```python
from build123d import *

# Parameters (mm, degrees)
SKETCH1_R           = 3
BOSS_EXTRUDE1_DEPTH = 54
SKETCH2_R           = 3
BOSS_EXTRUDE2_DEPTH = 35.293714059
SKETCH3_R           = 3
BOSS_EXTRUDE3_DEPTH = 6
BOSS_EXTRUDE4_START = 6
SKETCH4_R           = 3
BOSS_EXTRUDE4_DEPTH = 6


with BuildPart() as part:
    # Sketch1 → Boss-Extrude1 (new body)
    with BuildSketch(Plane(origin=(0, 0, 0), x_dir=(1, 0, 0), z_dir=(0, 1, 0))):
        with Locations(Location((0, 0, 0), (0, 0, 270))):
            Circle(SKETCH1_R)
    extrude(amount=BOSS_EXTRUDE1_DEPTH)

    # Sketch2 → Boss-Extrude2 (add)
    with BuildSketch(Plane(origin=(0, 54, 0), x_dir=(1, 0, 0), z_dir=(0, 1, 0))):
        with Locations(Location((0, 0, 0), (0, 0, 270))):
            Circle(SKETCH2_R)
    extrude(amount=BOSS_EXTRUDE2_DEPTH)

    # Sketch3 → Boss-Extrude3 (add)
    with BuildSketch(Plane(origin=(0, 89.293714059, 0), x_dir=(1, 0, 0), z_dir=(0, 1, 0))):
        with Locations(Location((0, 0, 0), (0, 0, 270))):
            Circle(SKETCH3_R)
    extrude(amount=BOSS_EXTRUDE3_DEPTH)

    # Sketch4 → Boss-Extrude4 (add)
    with BuildSketch(Plane.XZ.offset(BOSS_EXTRUDE4_START)):
        with Locations(Location((0, 0, 0), (0, 0, 270))):
            Circle(SKETCH4_R)
    extrude(amount=-BOSS_EXTRUDE4_DEPTH)


solid = part.part
```
Check sheet for the modelled part. Datum: model origin and axes. Units: mm. Give positions to 0.01 mm unless a question says otherwise; leave off trailing zeros. Loops run counter-clockwise (first coordinate to the right, second up) from the corner with the lowest first, then second, coordinate; pieces in that order, holes last. Notation, with made-up numbers: M 75,48 L 124,48 A23 cw 124,86 Z; hole C 27,-26.5 d7. An arc over 180 degrees is marked long. Answer as CSV lines item,"result".
Item 1: Scan lines: L1, parallel to Z at x = 0.1, y = 38; L2, parallel to Z at x = 1.15, y = 64.5; L3, parallel to X at y = 48, z = 0.55. Record each from-to range of solid material in increasing order.
Reply:
L1,"-3 to 3"
L2,"-2.77 to 2.77"
L3,"-2.95 to 2.95"
Item 2: Sectioned sample at A-A, the plane y = 65. Enter the section's corners in (x, z).
Reply:
outline,"C 0,0 d6"
Item 3: Depth check by flat-ended pin: pin 1 Ø1.5 at (x, y) = (-2, 40) entering from +Z. Enter the tip coordinate at first touch or a pass-through.
Reply:
pin 1,"z = 2.73"
Item 4: Sectioned sample at C-C, the plane x = -2.05. Enter the section's corners in (y, z).
Reply:
outline,"M -6,-2.19 L 95.29,-2.19 L 95.29,2.19 L -6,2.19 Z"
Item 5: Sectioned sample at B-B, the plane z = 1.85. Enter the section's corners in (x, y).
Reply:
outline,"M -2.36,-6 L 2.36,-6 L 2.36,95.29 L -2.36,95.29 Z"
